Here's how the part is built. I have some questions about the finished solid (model axes, mm). Face numbers are marked on the shaded views. A direction names the side the tool comes from. Coordinates: 2 decimals unless noted, no trailing zeros. Loops run counter-clockwise (first coordinate to the right, second up) from the corner with the lowest first, then second, coordinate; pieces in that order, holes last. Notation, with made-up numbers: M -33,3 L 12,3 A27 ccw 12,21 Z; hole C 78.25,-35 d7. An arc over 180 degrees is marked long. Use CSV: the item, a comma, the result in double quotes. Start each with the question number.
Q1. If we section it at B-B (x = 0): Please give me the cut outline in (y, z), and give its area (3 significant figures).
Q2. If we section it at D-D (z = -2.45): Please give me the cut outline in (x, y).
Q3. If we section it at C-C (y = 0.75): Please give me the cut outline in (x, z), and give its area (3 significant figures).
Q4. If we section it at A-A (y = -2): Please give me the cut outline in (x, z), and give its area (3 significant figures).
Q5. Please list where these lines run through material, in increasing order: probe 1 along Y at (x, z) = (0.55, -1.05); probe 2 along Y at (x, z) = (1.5, -2.55); probe 3 along X at (y, z) = (3.5, 0.6). Write a range as [from, to].
Q6. Which directions (+Z, -Z, +X, -X, +Y, -Y) give clear straight access to the entire face, cutting with the end or side of a thin tool? Please do the marked faces 4, 5 and 6.
Q7. If we mould it in two halves opening along X, with no side actions, what happens to the marked faces 1, 2 and 3? For each: +X half, -X half, draft (parallel to the pull), parting line (faces both ways), or undercut.
Q8. For pin 1 Ø1.5 at (x, y) = (1, -1.5) entering from -Z; pin 2 Ø0.9 at (x, y) = (0, -1.5) entering from -Z; pin 3 Ø0.5 at (x, y) = (0.5, -2) entering from +Z, each with a flat end and sliding along its axis, tell me the tip position at first contact or that it passes through.
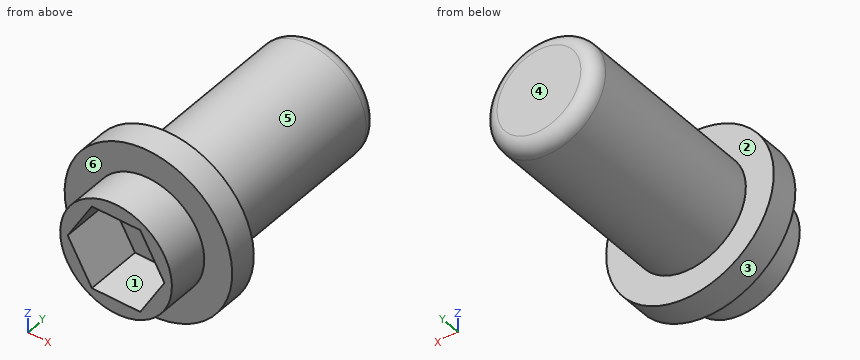
from build123d import *

# Parameters (mm, degrees)
SKETCH_1_R          = 2
EXTRUDE_1_DEPTH     = 7
FILLET_2_R          = 0.5
SKETCH_4_R          = 3
EXTRUDE_2_DEPTH     = 1
EXTRUDE_START       = 1.5
SKETCH_5_R          = 2
EXTRUDE_3_DEPTH     = 1.5
CUT_EXTRUDE_1_DEPTH = 2


with BuildPart() as part:
    # 草图1 → 凸台-拉伸1 (new body)
    with BuildSketch(Plane(origin=(0, 0, 0), x_dir=(1, 0, 0), z_dir=(0, 1, 0))):
        with Locations(Location((0, 0, 0), (0, 0, 270))):
            Circle(SKETCH_1_R)
    extrude(amount=EXTRUDE_1_DEPTH)

    # 圆角2
    fillet_2_edges = [part.edges().sort_by_distance(p)[0] for p in [
        (0, 7, -2),
    ]]
    fillet(fillet_2_edges, radius=FILLET_2_R)

    # 草图4 → 凸台-拉伸2 (add)
    with BuildSketch(Plane.XZ):
        with Locations(Location((0, 0, 0), (0, 0, 270))):
            Circle(SKETCH_4_R)
    extrude(amount=EXTRUDE_2_DEPTH)

    # 草图5 → 凸台-拉伸3 (add)
    with BuildSketch(Plane.XZ.offset(1).offset(EXTRUDE_START)):
        with Locations(Location((0, 0, 0), (0, 0, 90))):
            Circle(SKETCH_5_R)
    extrude(amount=-EXTRUDE_3_DEPTH)

    # 草图6 → 切除-拉伸1 (cut)
    with BuildSketch(Plane.XZ.offset(2.5)):
        Polygon((1.732050808, 0), (0.866025404, 1.5), (-0.866025404, 1.5), (-1.732050808, 0), (-0.866025404, -1.5), (0.866025404, -1.5), align=None)
    extrude(amount=-CUT_EXTRUDE_1_DEPTH, mode=Mode.SUBTRACT)


solid = part.part
Results below:
1,outline,"M -2.5,-2 L -1,-2 L -1,-3 L 0,-3 L 0,-2 L 6.5,-2 A0.5 ccw 7,-1.5 L 7,1.5 A0.5 ccw 6.5,2 L 0,2 L 0,3 L -1,3 L -1,2 L -2.5,2 L -2.5,1.5 L -0.5,1.5 L -0.5,-1.5 L -2.5,-1.5 Z"
1,area,"33.9 mm^2"
2,outline,"M -1.73,-1 L 1.73,-1 L 1.73,0 L -1.73,0 Z"
3,outline,"C 0,0 d4"
3,area,"12.6 mm^2"
4,outline,"C 0,0 d4; hole M -1.73,0 L -0.87,-1.5 L 0.87,-1.5 L 1.73,0 L 0.87,1.5 L -0.87,1.5 Z"
4,area,"4.77 mm^2"
5,probe 1,"[-0.5, 7]"
5,probe 2,"[-1, 0]"
5,probe 3,"[-1.91, 1.91]"
6,face 4,"+Z, -Z, +X, -X, +Y"
6,face 5,"+Y"
6,face 6,"-Y"
7,face 1,"undercut"
7,face 2,"draft"
7,face 3,"parting line"
8,pin 1,"z = -2.97"
8,pin 2,"z = -2"
8,pin 3,"z = 1.98"
